from build123d import *

# Parameters (mm, degrees)
OUTER_SHAPE_DEPTH  = 4
MIDDLE_WALL_DEPTH  = 0.1
HOLES_R            = 3.1
OUTER_HOLE_DEPTH   = 3.9
SKETCH3_R          = 3.1
SKETCH3_R_2        = 2.4
INNER_HOLE_DEPTH   = 3.1
SKETCH4_R          = 2.4
THROUGH_HOLE_DEPTH = 5


with BuildPart() as part:
    # Sketch1 → Outer Shape (new body)
    with BuildSketch(Plane.XY):
        with BuildLine():
            Line((-16.421445021, 3.7), (16.421445021, 3.7))
            ThreePointArc((16.421445021, 3.7), (20.121445021, 0), (16.421445021, -3.7))
            Line((16.421445021, -3.7), (-16.421445021, -3.7))
            ThreePointArc((-16.421445021, -3.7), (-20.121445021, 0), (-16.421445021, 3.7))
        make_face()
        with BuildLine():
            Line((-16, 3.1), (16, 3.1))
            ThreePointArc((16, 3.1), (19.1, 0), (16, -3.1))
            Line((16, -3.1), (-16, -3.1))
            ThreePointArc((-16, -3.1), (-19.1, 0), (-16, 3.1))
        make_face(mode=Mode.SUBTRACT)
    extrude(amount=OUTER_SHAPE_DEPTH)



with BuildPart() as body_2:
    # Sketch2 → Middle wall (new body)
    with BuildSketch(Plane.XY):
        with BuildLine():
            Line((-15.918927506, 3.189649288), (15.918927506, 3.189649288))
            ThreePointArc((15.918927506, 3.189649288), (19.108576794, 0), (15.918927506, -3.189649288))
            Line((15.918927506, -3.189649288), (-15.918927506, -3.189649288))
            ThreePointArc((-15.918927506, -3.189649288), (-19.108576794, 0), (-15.918927506, 3.189649288))
        make_face()
    extrude(amount=MIDDLE_WALL_DEPTH)


with BuildPart() as part_1:
    add(part.part)

    add(body_2.part)  # Outer Hole merges body 2
    # Holes → Outer Hole (add)
    with BuildSketch(Plane.XY.offset(0.1)):
        with BuildLine():
            Line((-6.12486336, 3.189649288), (-9.87513664, 3.189649288))
            ThreePointArc((-9.87513664, 3.189649288), (-11.7, 0), (-9.87513664, -3.189649288))
            Line((-9.87513664, -3.189649288), (-6.12486336, -3.189649288))
            ThreePointArc((-6.12486336, -3.189649288), (-4.788457881, -1.837388695), (-4.3, 0))
            ThreePointArc((-4.3, 0), (-4.788457881, 1.837388695), (-6.12486336, 3.189649288))
        make_face()
        with Locations((-8, 0)):
            Circle(HOLES_R, mode=Mode.SUBTRACT)
        with BuildLine():
            ThreePointArc((-14.12486336, -3.189649288), (-12.788457881, -1.837388695), (-12.3, 0))
            ThreePointArc((-12.3, 0), (-12.788457881, 1.837388695), (-14.12486336, 3.189649288))
            Line((-14.12486336, 3.189649288), (-15.918927506, 3.189649288))
            ThreePointArc((-15.918927506, 3.189649288), (-19.108576794, 0), (-15.918927506, -3.189649288))
            Line((-15.918927506, -3.189649288), (-14.12486336, -3.189649288))
        make_face()
        with Locations((-16, 0)):
            Circle(HOLES_R, mode=Mode.SUBTRACT)
        with BuildLine():
            Line((1.87513664, 3.189649288), (-1.87513664, 3.189649288))
            ThreePointArc((-1.87513664, 3.189649288), (-3.7, 0), (-1.87513664, -3.189649288))
            Line((-1.87513664, -3.189649288), (1.87513664, -3.189649288))
            ThreePointArc((1.87513664, -3.189649288), (3.211542119, -1.837388695), (3.7, 0))
            ThreePointArc((3.7, 0), (3.211542119, 1.837388695), (1.87513664, 3.189649288))
        make_face()
        Circle(HOLES_R, mode=Mode.SUBTRACT)
        with BuildLine():
            Line((9.87513664, 3.189649288), (6.12486336, 3.189649288))
            ThreePointArc((6.12486336, 3.189649288), (4.3, 0), (6.12486336, -3.189649288))
            Line((6.12486336, -3.189649288), (9.87513664, -3.189649288))
            ThreePointArc((9.87513664, -3.189649288), (11.211542119, -1.837388695), (11.7, 0))
            ThreePointArc((11.7, 0), (11.211542119, 1.837388695), (9.87513664, 3.189649288))
        make_face()
        with Locations((8, 0)):
            Circle(HOLES_R, mode=Mode.SUBTRACT)
        with BuildLine():
            Line((15.918927506, 3.189649288), (14.12486336, 3.189649288))
            ThreePointArc((14.12486336, 3.189649288), (12.3, 0), (14.12486336, -3.189649288))
            Line((14.12486336, -3.189649288), (15.918927506, -3.189649288))
            ThreePointArc((15.918927506, -3.189649288), (19.108576794, 0), (15.918927506, 3.189649288))
        make_face()
        with Locations((16, 0)):
            Circle(HOLES_R, mode=Mode.SUBTRACT)
    extrude(amount=OUTER_HOLE_DEPTH)

    # Sketch3 → Inner Hole (add)
    with BuildSketch(Plane.XY):
        with Locations((-16, 0)):
            Circle(SKETCH3_R)
        with Locations((-16, 0)):
            Circle(SKETCH3_R_2, mode=Mode.SUBTRACT)
        with Locations((-8, 0)):
            Circle(SKETCH3_R)
        with Locations((-8, 0)):
            Circle(SKETCH3_R_2, mode=Mode.SUBTRACT)
        Circle(SKETCH3_R)
        Circle(SKETCH3_R_2, mode=Mode.SUBTRACT)
        with Locations((8, 0)):
            Circle(SKETCH3_R)
        with Locations((8, 0)):
            Circle(SKETCH3_R_2, mode=Mode.SUBTRACT)
        with Locations((16, 0)):
            Circle(SKETCH3_R)
        with Locations((16, 0)):
            Circle(SKETCH3_R_2, mode=Mode.SUBTRACT)
    extrude(amount=INNER_HOLE_DEPTH)

    # Sketch4 → Through Hole (cut, through all)
    with BuildSketch(Plane.XY):
        with Locations((-16, 0)):
            Circle(SKETCH4_R)
        with Locations((-8, 0)):
            Circle(SKETCH4_R)
        Circle(SKETCH4_R)
        with Locations((8, 0)):
            Circle(SKETCH4_R)
        with Locations((16, 0)):
            Circle(SKETCH4_R)
    extrude(amount=THROUGH_HOLE_DEPTH, mode=Mode.SUBTRACT)

    # Mirror1: part across face


with BuildPart() as part_2:
    add(part_1.part)
    add(part_1.part.mirror(Plane(origin=(0, 0, 0), x_dir=(1, 0, 0), z_dir=(0, 0, -1))))


solid = part_2.part
For this review, take the finished solid that the model builds, in its own axes (mm). A direction names the side the tool comes from. Round coordinates to 2 decimals unless told otherwise and drop trailing zeros. Write each loop counter-clockwise with the first axis right and the second up, starting at its lowest first coordinate (ties: lowest second). Pieces come first, ordered by that corner, then holes. Notation, with made-up numbers: (83, -22) -> (100, -22) arc R19 ccw to (100, 6) -> close; hole circle Ø8 at (22, -24.75). An arc over 180 degrees is marked (long way). Put each result on its own line as item: value.
Q1. The part is to be moulded in two halves that separate along X. For faces 1 (the flat face through (3.1, 1.4, 4)), 2 (the flat face through (-4, 3.1, -2)), say which applies: released by +X, released by -X, zero draft, split by the parting line, or undercut.
Determined:
face 1: zero draft
face 2: undercut
Q2. Consider section D-D on x = -1.5. State the section outline as (y, z) points, and give its area (3 significant figures).
Determined:
outline: (-3.7, -4) -> (-2.71, -4) -> (-2.71, -3.1) -> (-1.87, -3.1) -> (-1.87, 3.1) -> (-2.71, 3.1) -> (-2.71, 4) -> (-3.7, 4) -> close; (1.87, -3.1) -> (2.71, -3.1) -> (2.71, -4) -> (3.7, -4) -> (3.7, 4) -> (2.71, 4) -> (2.71, 3.1) -> (1.87, 3.1) -> close
area: 26.2 mm^2
Q3. Consider section A-A on z = 0.75. Give the number of separate pieces and of enclosed holes in the cut face, and give its area (3 significant figures).
Determined:
separate pieces: 1
enclosed holes: 9
area: 156 mm^2
Q4. Machinability: for faces 3 (the flat face through (-12, 0, 0.1)), 4 (the flat face through (-4, 0, -0.1)), which of the approach directions +Z, -Z, +X, -X, +Y, -Y give a long, thin tool a straight path to every point of the face, cutting with its end or side? Answer none if there is none.
Determined:
face 3: +Z
face 4: -Z
Q5. To check wall thickness, follow L1, parallel to X at y = 2.5, z = -0.25; L2, parallel to X at y = -3, z = -2.25; L3, parallel to Y at x = 13.5, z = -1.25. State the ranges of each line that lie inside material, in increasing order. Write a range as [from, to].
Determined:
L1: x = [-19.15, -13.27], [-10.73, -5.27], [-2.73, 2.73], [5.27, 10.73], [13.27, 19.15]
L2: x = [-18.59, -13.83], [-10.17, -5.83], [-2.17, 2.17], [5.83, 10.17], [13.83, 18.59]
L3: y = [-3.7, -3.1], [-2.73, 2.73], [3.1, 3.7]
Q6. Consider section B-B on x = 15. State the section outline as (y, z) points.
Determined:
outline: (-3.7, -4) -> (-2.93, -4) -> (-2.93, -3.1) -> (-2.18, -3.1) -> (-2.18, 3.1) -> (-2.93, 3.1) -> (-2.93, 4) -> (-3.7, 4) -> close; (2.18, -3.1) -> (2.93, -3.1) -> (2.93, -4) -> (3.7, -4) -> (3.7, 4) -> (2.93, 4) -> (2.93, 3.1) -> (2.18, 3.1) -> close
Q7. Clearance check with a flat-ended pin moving along its axis: pin 1 Ø1 at (y, z) = (2.5, -2.5) entering from +X. State where the tip first meets the part, or that it passes through.
Determined:
pin 1: stops at x = 19.53
